Here's how the part is built. I have some questions about the finished solid (model axes, mm). Face numbers are marked on the shaded views. A direction names the side the tool comes from. Give positions to 0.01 mm unless a question says otherwise; leave off trailing zeros. Write each loop counter-clockwise with the first axis right and the second up, starting at its lowest first coordinate (ties: lowest second). Pieces come first, ordered by that corner, then holes. Notation, with made-up numbers: (25.5, -37) - (31.5, -37) arc R14 ccw to (31.5, -13) - close; hole circle Ø2 at (77, 43.25). An arc over 180 degrees is marked (long way). Write each question's results on one line, items separated by ' | '. Start each with the question number.
Item 1: Suppose I cut it at C-C on y = 363. List the corners of the cut face in (x, z) for me, then the cut area to 3 significant figures.
Item 2: Will these pins go through, and if not, where does the flat tip stop? P1, Ø10, axis at x = 173.5, y = 302.5, coming from the -Z side; P2, Ø2, axis at x = 177, y = 363.5, coming from the -Z side; P3, Ø1, axis at x = 106.5, y = 984.5, coming from the -Z side.
Item 3: Which directions (+Z, -Z, +X, -X, +Y, -Y) give clear straight access to the entire face, cutting with the end or side of a thin tool? Please do the marked faces 4, 5, 6 and 7.
Item 4: We'd pull the mould along Y, two halves only. Please class the marked faces 1, 2 and 3: +Y half, -Y half, draft (parallel to the pull), parting line (faces both ways), or undercut.
Item 5: Suppose I cut it at B-B on x = 37.5. List the corners of the cut face in (y, z) for me, then the cut area to 3 significant figures.
Item 6: Please list where these lines run through material, in increasing order: line 1 along Y through (x, z) = (277.5, -119.5); line 2 along Z through (x, y) = (153, 801); line 3 along Y through (x, z) = (223.5, -652).
Item 7: Suppose I cut it at A-A on z = -327. List the corners of the cut face in (x, y) for me.
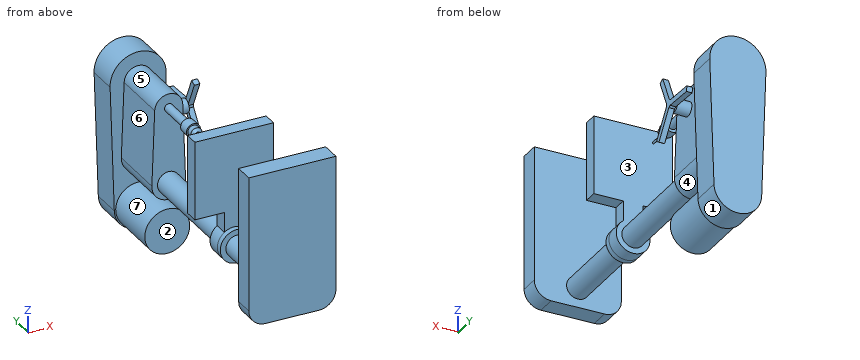
```python
from build123d import *

# Parameters (mm, degrees)
SKETCH_1_W          = 310
SKETCH_1_H          = 540
EXTRUDE_1_DEPTH     = 70
FILLET_1_R          = 60
SKETCH_2_R          = 40
EXTRUDE_2_DEPTH     = 310
SKETCH_3_R          = 60
EXTRUDE_3_DEPTH     = 20
EXTRUDE_4_DEPTH     = 50
SKETCH_5_R          = 40
EXTRUDE_5_DEPTH     = 400
EXTRUDE_6_DEPTH     = 210
EXTRUDE_7_DEPTH     = 110
SKETCH_10_R         = 80
EXTRUDE_8_DEPTH     = 200
SKETCH_11_R         = 15
EXTRUDE_9_DEPTH     = 130
SKETCH_12_R         = 25
EXTRUDE_10_DEPTH    = 40
SKETCH_13_R         = 20
EXTRUDE_11_DEPTH    = 30
CHAMFER_1_SIZE      = 10
SKETCH_14_R         = 3.5
EXTRUDE_12_DEPTH    = 60
SKETCH_15_R         = 25
EXTRUDE_13_DEPTH    = 50
SKETCH_16_R         = 125
EXTRUDE_14_DEPTH    = 20
CUT_EXTRUDE_START   = -20
CUT_EXTRUDE_1_DEPTH = 20


with BuildPart() as part:
    # ｽｹｯﾁ1 → ﾎﾞｽ - 押し出し1 (new body)
    with BuildSketch(Plane(origin=(0, 0, 0), x_dir=(1, 0, 0), z_dir=(0, 1, 0))):
        with Locations((155, 270)):
            Rectangle(SKETCH_1_W, SKETCH_1_H)
    extrude(amount=EXTRUDE_1_DEPTH)

    # ﾌｨﾚｯﾄ1
    fillet_1_edges = [part.edges().sort_by_distance(p)[0] for p in [
        (0, 35, -540),
        (310, 35, -540),
    ]]
    fillet(fillet_1_edges, radius=FILLET_1_R)

    # ｽｹｯﾁ2 → ﾎﾞｽ - 押し出し2 (add)
    with BuildSketch(Plane(origin=(0, 70, 0), x_dir=(1, 0, 0), z_dir=(0, 1, 0))):
        with Locations(Location((155, 470, 0), (0, 0, 90))):
            Circle(SKETCH_2_R)
    extrude(amount=EXTRUDE_2_DEPTH)

    # ｽｹｯﾁ3 → ﾎﾞｽ - 押し出し3 (add)
    with BuildSketch(Plane(origin=(0, 380, 0), x_dir=(1, 0, 0), z_dir=(0, 1, 0))):
        with Locations(Location((155, 470, 0), (0, 0, 270))):
            Circle(SKETCH_3_R)
    extrude(amount=EXTRUDE_3_DEPTH)

    # ｽｹｯﾁ4 → ﾎﾞｽ - 押し出し4 (add)
    with BuildSketch(Plane(origin=(0, 400, 0), x_dir=(1, 0, 0), z_dir=(0, 1, 0))):
        with BuildLine():
            Line((190, 350), (295, 350))
            Line((295, 350), (295, 70))
            Line((295, 70), (15, 70))
            Line((15, 70), (15, 350))
            Line((15, 350), (120, 350))
            Line((120, 350), (120, 421.266028276))
            ThreePointArc((120, 421.266028276), (155, 530), (190, 421.266028276))
            Line((190, 421.266028276), (190, 350))
        make_face()
    extrude(amount=EXTRUDE_4_DEPTH)

    # ｽｹｯﾁ5 → ﾎﾞｽ - 押し出し5 (add)
    with BuildSketch(Plane(origin=(0, 450, 0), x_dir=(1, 0, 0), z_dir=(0, 1, 0))):
        with Locations(Location((155, 470, 0), (0, 0, 90))):
            Circle(SKETCH_5_R)
    extrude(amount=EXTRUDE_5_DEPTH)

    # ｽｹｯﾁ8 → ﾎﾞｽ - 押し出し6 (add)
    with BuildSketch(Plane(origin=(0, 850, 0), x_dir=(1, 0, 0), z_dir=(0, 1, 0))):
        with BuildLine():
            Line((95.041166386, 467.777777778), (105.034305321, 198.148148148))
            ThreePointArc((105.034305321, 198.148148148), (155, 150), (204.965694679, 198.148148148))
            Line((204.965694679, 198.148148148), (214.958833614, 467.777777778))
            ThreePointArc((214.958833614, 467.777777778), (155, 530), (95.041166386, 467.777777778))
        make_face()
    extrude(amount=EXTRUDE_6_DEPTH)

    # ｽｹｯﾁ9 → ﾎﾞｽ - 押し出し7 (add)
    with BuildSketch(Plane(origin=(0, 1060, 0), x_dir=(1, 0, 0), z_dir=(0, 1, 0))):
        with BuildLine():
            Line((55.055570996, 203.333333333), (70.047235347, 652.833333333))
            ThreePointArc((70.047235347, 652.833333333), (155, 735), (239.952764653, 652.833333333))
            Line((239.952764653, 652.833333333), (254.944429004, 203.333333333))
            ThreePointArc((254.944429004, 203.333333333), (155, 100), (55.055570996, 203.333333333))
        make_face()
    extrude(amount=EXTRUDE_7_DEPTH)

    # ｽｹｯﾁ10 → ﾎﾞｽ - 押し出し8 (add)
    with BuildSketch(Plane(origin=(0, 1060, 0), x_dir=(-1, 0, 0), z_dir=(0, -1, 0))):
        with Locations(Location((-155, 650, 0), (0, 0, 270))):
            Circle(SKETCH_10_R)
    extrude(amount=EXTRUDE_8_DEPTH)

    # ｽｹｯﾁ11 → ﾎﾞｽ - 押し出し9 (add)
    with BuildSketch(Plane(origin=(0, 850, 0), x_dir=(-1, 0, 0), z_dir=(0, -1, 0))):
        with Locations(Location((-155, 200, 0), (0, 0, 270))):
            Circle(SKETCH_11_R)
    extrude(amount=EXTRUDE_9_DEPTH)

    # ｽｹｯﾁ12 → ﾎﾞｽ - 押し出し10 (add)
    with BuildSketch(Plane(origin=(0, 720, 0), x_dir=(-1, 0, 0), z_dir=(0, -1, 0))):
        with Locations(Location((-155, 200, 0), (0, 0, 90))):
            Circle(SKETCH_12_R)
    extrude(amount=EXTRUDE_10_DEPTH)

    # ｽｹｯﾁ13 → ﾎﾞｽ - 押し出し11 (add)
    with BuildSketch(Plane(origin=(0, 680, 0), x_dir=(-1, 0, 0), z_dir=(0, -1, 0))):
        with Locations(Location((-155, 200, 0), (0, 0, 90))):
            Circle(SKETCH_13_R)
    extrude(amount=EXTRUDE_11_DEPTH)

    # 面取り1
    chamfer_1_edges = [part.edges().sort_by_distance(p)[0] for p in [
        (155, 650, -180),
    ]]
    chamfer(chamfer_1_edges, length=CHAMFER_1_SIZE)

    # ｽｹｯﾁ14 → ﾎﾞｽ - 押し出し12 (add)
    with BuildSketch(Plane(origin=(0, 650, 0), x_dir=(-1, 0, 0), z_dir=(0, -1, 0))):
        with Locations(Location((-155, 200, 0), (0, 0, 90))):
            Circle(SKETCH_14_R)
    extrude(amount=EXTRUDE_12_DEPTH)

    # ｽｹｯﾁ15 → ﾎﾞｽ - 押し出し13 (add)
    with BuildSketch(Plane(origin=(197.350749514, 0, 7.314305411), x_dir=(0.0370370370370371, 0, -0.9993138935727439), z_dir=(0.9993138935727439, 0, 0.0370370370370371))):
        with Locations(Location((265.603519455, 930, 0), (0, 0, 180))):
            Circle(SKETCH_15_R)
    extrude(amount=EXTRUDE_13_DEPTH)

    # ｽｹｯﾁ16 → ﾎﾞｽ - 押し出し14 (add)
    with BuildSketch(Plane(origin=(247.316444192, 0, 9.166157263), x_dir=(0.03703703703703711, 0, -0.9993138935727439), z_dir=(0.9993138935727439, 0, 0.03703703703703711))):
        with Locations((265.603519455, 930)):
            Circle(SKETCH_16_R)
    extrude(amount=EXTRUDE_14_DEPTH)

    # ｽｹｯﾁ17 → ｶｯﾄ - 押し出し1 (cut)
    with BuildSketch(Plane(origin=(267.302722064, 0, 9.906898004), x_dir=(0.037037037037037125, 0, -0.9993138935727439), z_dir=(0.9993138935727439, 0, 0.037037037037037125)).offset(CUT_EXTRUDE_START)):
        with BuildLine():
            Line((150.427943116, 881.424423678), (251.071784865, 933.718694636))
            ThreePointArc((251.071784865, 933.718694636), (252.958803035, 938.069147828), (256.109578031, 941.613142393))
            Line((256.109578031, 941.613142393), (261.143331784, 1054.92040156))
            ThreePointArc((261.143331784, 1054.92040156), (160.230882623, 997.242898563), (150.427943116, 881.424423678))
        make_face()
        with BuildLine():
            ThreePointArc((390.603519455, 930), (359.318547956, 1012.719365526), (281.123624526, 1054.032763166))
            Line((281.123624526, 1054.032763166), (276.089870774, 940.725503999))
            ThreePointArc((276.089870774, 940.725503999), (278.913964671, 936.916071729), (280.407766497, 932.415423259))
            Line((280.407766497, 932.415423259), (376.017854493, 871.402435049))
            ThreePointArc((376.017854493, 871.402435049), (386.90230733, 899.80721841), (390.603519455, 930))
        make_face()
        with BuildLine():
            Line((260.293213837, 915.971434348), (159.649372089, 863.677163391))
            ThreePointArc((159.649372089, 863.677163391), (260.055779492, 805.123170359), (365.258990723, 854.542813156))
            Line((365.258990723, 854.542813156), (269.648902727, 915.555801366))
            ThreePointArc((269.648902727, 915.555801366), (264.93779066, 915.014780443), (260.293213837, 915.971434348))
        make_face()
    extrude(amount=CUT_EXTRUDE_1_DEPTH, mode=Mode.SUBTRACT)


solid = part.part
```
Checked values:
1) outline: circle Ø80 at (155, -470) | area: 5,030 mm^2
2) P1: stops at z = -507.65 | P2: stops at z = -504.04 | P3: stops at z = -714
3) face 4: none | face 5: +Z | face 6: +Z, -X | face 7: -Y
4) face 1: draft | face 2: -Y half | face 3: undercut
5) outline: (0, -535.62) - (70, -535.62) - (70, 0) - (0, 0) - close; (400, -350) - (450, -350) - (450, -70) - (400, -70) - close | area: 51,500 mm^2
6) line 1: y = 0 to 70, 400 to 450 | line 2: z = -509.95 to -430.05, -214.87 to -185.13 | line 3: y = 860 to 1170
7) outline: (0, 0) - (310, 0) - (310, 70) - (0, 70) - close; (15, 400) - (295, 400) - (295, 450) - (15, 450) - close; (59.18, 1060) - (100.26, 1060) - (100.26, 850) - (209.74, 850) - (209.74, 1060) - (250.82, 1060) - (250.82, 1170) - (59.18, 1170) - close; (259.78, 872.96) - (279.79, 872.49) - (279.79, 896.21) - (259.78, 896.69) - close
